```python
from build123d import *

# Parameters (mm, degrees)
ESQUISSE1_R             = 7.5
BOSS_EXTRU_1_DEPTH      = 30
ESQUISSE4_R             = 1.6
ENL_V_MAT_EXTRU_2_DEPTH = 32.819805295
ESQUISSE5_W             = 2
ESQUISSE5_H             = 2.6861835
ENL_V_MAT_EXTRU_3_DEPTH = 32.819805295


with BuildPart() as part:
    # Esquisse1 → Boss.-Extru.1 (new body)
    with BuildSketch(Plane(origin=(0, 0, 0), x_dir=(0, 0, -1), z_dir=(1, 0, 0))):
        Circle(ESQUISSE1_R)
    extrude(amount=BOSS_EXTRU_1_DEPTH)

    # Enlèv. mat.-Extru.1 cone 1 section (through the dimple's axis) → Enlèv. mat.-Extru.1 (revolve, cut)
    with BuildSketch(Plane(origin=(9.5, 0, 7.5), x_dir=(0, -1, 0), z_dir=(1, 0, 0))):
        Polygon((0, 0), (2.5, 0), (0, 4.330127019), align=None)
    revolve(axis=Axis((9.5, 0, 7.5), (0, 0, -1)), mode=Mode.SUBTRACT)

    # Esquisse4 → Enlèv. mat.-Extru.2 (cut, through all)
    with BuildSketch(Plane.ZY):
        Circle(ESQUISSE4_R)
    extrude(amount=-ENL_V_MAT_EXTRU_2_DEPTH, mode=Mode.SUBTRACT)

    # Esquisse5 → Enlèv. mat.-Extru.3 (cut, through all)
    with BuildSketch(Plane(origin=(30, 0, 0), x_dir=(0, 0, -1), z_dir=(1, 0, 0))):
        with Locations((0, 6.84309175)):
            Rectangle(ESQUISSE5_W, ESQUISSE5_H)
        with Locations((0, -6.84309175)):
            Rectangle(ESQUISSE5_W, ESQUISSE5_H)
    extrude(amount=-ENL_V_MAT_EXTRU_3_DEPTH, mode=Mode.SUBTRACT)


solid = part.part
```
Input: part model. Units: mm. Frame: model coordinates. A direction names the side the tool comes from. Coordinates: 2 decimals unless noted, no trailing zeros. Loops run counter-clockwise (first coordinate to the right, second up) from the corner with the lowest first, then second, coordinate; pieces in that order, holes last. Notation, with made-up numbers: (29, 11) -> (65, 11) arc R26 cw to (65, 27) -> close; hole circle Ø11 at (2, -32). An arc over 180 degrees is marked (long way). Use a Markdown table: item, result.
1) Cut plane B-B (x = 18.5). Return the cut outline in (y, z), then the cut area to 3 significant figures.
Results found:
| item | result |
|---|---|
| outline | (-7.43, -1) arc R7.5 ccw to (7.43, -1) -> (5.5, -1) -> (5.5, 1) -> (7.43, 1) arc R7.5 ccw to (-7.43, 1) -> (-5.5, 1) -> (-5.5, -1) -> close; hole circle Ø3.2 at (0, 0) |
| area | 161 mm2 |
2) Access query for faces 1 (the cylindrical face through (14.79, -0.15, -7.5)), 2 (the flat face through (15, -5.5, 0)), 3 (the flat face through (15, 5.5, 0)). Directions: +Z, -Z, +X, -X, +Y, -Y. A direction counts if a zero-diameter tool reaches every point of the face in a straight line with its end or side. Return the directions, or none.
Results found:
| item | result |
|---|---|
| face 1 | -Z, +X, -X |
| face 2 | +X, -X, -Y |
| face 3 | +X, -X, +Y |
3) Cut plane A-A (z = 0). Return the cut outline in (x, y), then the cut area to 3 significant figures.
Results found:
| item | result |
|---|---|
| outline | (0, -5.5) -> (30, -5.5) -> (30, -1.6) -> (0, -1.6) -> close; (0, 1.6) -> (30, 1.6) -> (30, 5.5) -> (0, 5.5) -> close |
| area | 234 mm2 |
4) Cut plane D-D (y = -3.25). Return the cut outline in (x, z), then the cut area to 3 significant figures.
Results found:
| item | result |
|---|---|
| outline | (0, -6.76) -> (30, -6.76) -> (30, 6.76) -> (0, 6.76) -> close |
| area | 406 mm2 |
5) Cut plane C-C (z = 6). Return the cut outline in (x, y).
Results found:
| item | result |
|---|---|
| outline | (0, -4.5) -> (30, -4.5) -> (30, 4.5) -> (0, 4.5) -> close; hole circle Ø3.27 at (9.5, 0) |
6) Contact query for flat-ended pins moving along their axis: pin 1 (4 mm diameter, centred on x = 12.5, z = -5, fed in from -Y); pin 2 (1.5 mm diameter, centred on x = 8, y = -7, fed in from +Z); pin 3 (1.5 mm diameter, centred on x = 14, y = -6, fed in from -Z). Output: stop coordinate, or through.
Results found:
| item | result |
|---|---|
| pin 1 | stops at y = -6.87 |
| pin 2 | stops at z = 4.15 |
| pin 3 | stops at z = -5.36 |
7) Pull-direction query (X, two-part tool) for faces 4 (the flat face through (30, 2, 0)), 5 (the flat face through (15, -6, 1)), 6 (the conical face through (9.46, 0.95, 4.82)); classes: released by +X, released by -X, zero draft, split by the parting line, or undercut.
Results found:
| item | result |
|---|---|
| face 4 | released by +X |
| face 5 | zero draft |
| face 6 | undercut |
8) Material intervals for line 1 along Y through (x, z) = (11.5, 0); line 2 along Z through (x, y) = (28.5, -5.75); line 3 along Z through (x, y) = (2.5, -4), sorted ascending. Write a range as from..to.
Results found:
| item | result |
|---|---|
| line 1 | y = -5.5..-1.6, 1.6..5.5 |
| line 2 | z = -4.82..-1, 1..4.82 |
| line 3 | z = -6.34..6.34 |
